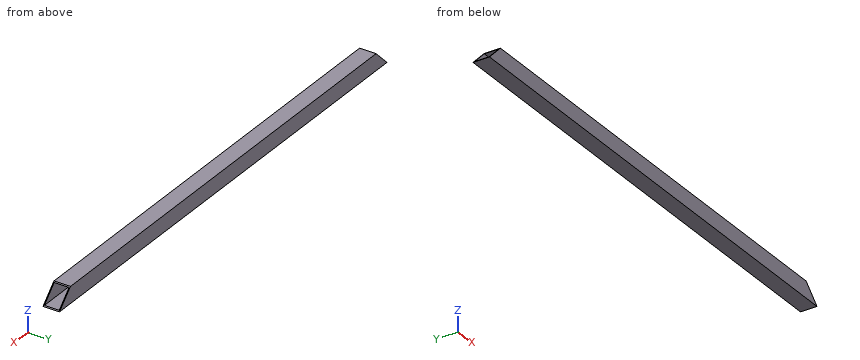
```python
from build123d import *

# Parameters (mm, degrees)
F0_W     = 1524
F0_H     = 50.8
F1_DEPTH = 50.8
F2_T     = -2.54
F4_DEPTH = 50.801
F6_DEPTH = 50.801


with BuildPart() as f1:
    # F0 (on Top) → F1 (new body)
    with BuildSketch(Plane.XY):
        Rectangle(F0_W, F0_H)
    extrude(amount=F1_DEPTH)

    # F2
    f2_openings = [f1.faces().sort_by_distance(p)[0] for p in [
        (-762, 0, 25.4),
        (762, 0, 25.4),
    ]]
    offset(amount=F2_T, openings=f2_openings)

    # F3 (on face) → F4 (cut, through all)
    with BuildSketch(Plane.XZ.offset(25.4)):
        Polygon((711.2, 50.8), (762, 0), (762, 50.8), align=None)
    extrude(amount=-F4_DEPTH, mode=Mode.SUBTRACT)

    # F5 (on face) → F6 (cut, through all)
    with BuildSketch(Plane.XZ.offset(25.4)):
        Polygon((-762, 50.8), (-762, 0), (-711.2, 50.8), align=None)
    extrude(amount=-F6_DEPTH, mode=Mode.SUBTRACT)


solid = f1.part
```
CAD build for the part. Positions are in the model's coordinates, mm. Give positions to 0.01 mm unless a question says otherwise; leave off trailing zeros. Write each loop counter-clockwise with the first axis right and the second up, starting at its lowest first coordinate (ties: lowest second). Pieces come first, ordered by that corner, then holes. Notation, with made-up numbers: M -25,76.5 L 2,76.5 A14 ccw 2,88.5 Z; hole C 62.5,86 d4. An arc over 180 degrees is marked long. Return JSON: item names as keys, results as strings. Group by question number.
(1) Band-saw the part on A-A (z = 16). Give the cut face in (x, y).
(2) Flat gauge pin, fed straight in: pin 1 Ø5 at (x, y) = (433.5, -6) entering from -Z. Where does the tip first touch, or does it go through?
(3) Band-saw the part on B-B (y = 13). Give the cut face in (x, z).
(4) Band-saw the part on C-C (x = 134). Give the cut face in (y, z), and give its area (3 significant figures).
(5) Drill centre lines: L1, parallel to Y at x = -377.5, z = 12.5; L2, parallel to Z at x = 641.5, y = 17.5; L3, parallel to X at y = -4, z = 48.5. Where is each one in solid material? Low to high. Write a range as [from, to].
Entries:
{
 "1": {"outline": "M -746,-25.4 L 746,-25.4 L 746,-22.86 L -746,-22.86 Z; M -746,22.86 L 746,22.86 L 746,25.4 L -746,25.4 Z"},
 "2": {"pin 1": "stops at z = 0"},
 "3": {"outline": "M -762,0 L 762,0 L 759.46,2.54 L -759.46,2.54 Z; M -713.74,48.26 L 713.74,48.26 L 711.2,50.8 L -711.2,50.8 Z"},
 "4": {"outline": "M -25.4,0 L 25.4,0 L 25.4,50.8 L -25.4,50.8 Z; hole M -22.86,2.54 L 22.86,2.54 L 22.86,48.26 L -22.86,48.26 Z", "area": "490 mm^2"},
 "5": {"L1": "y = [-25.4, -22.86], [22.86, 25.4]", "L2": "z = [0, 2.54], [48.26, 50.8]", "L3": "x = [-713.5, 713.5]"}
}
